```python
from build123d import *

# Parameters (mm, degrees)
SKETCH1_R           = 7.239
SKETCH1_R_2         = 2.15
SKETCH1_R_3         = 1.65
BOSS_EXTRUDE1_DEPTH = 3
FILLET1_R           = 10


with BuildPart() as part:
    # Sketch1 → Boss-Extrude1 (new body)
    with BuildSketch(Plane.XY):
        with BuildLine():
            Line((-87.4, 48.933577685), (87.4, 48.933577685))
            Line((87.4, 48.933577685), (97.4, 48.933577685))
            Line((97.4, 48.933577685), (138.294602876, 18.952308855))
            ThreePointArc((138.294602876, 18.952308855), (147.9, 0), (138.294602876, -18.952308855))
            Line((138.294602876, -18.952308855), (97.4, -48.933577685))
            Line((97.4, -48.933577685), (87.4, -48.933577685))
            Line((87.4, -48.933577685), (-87.4, -48.933577685))
            Line((-87.4, -48.933577685), (-97.4, -48.933577685))
            Line((-97.4, -48.933577685), (-138.294602876, -18.952308855))
            ThreePointArc((-138.294602876, -18.952308855), (-147.9, 0), (-138.294602876, 18.952308855))
            Line((-138.294602876, 18.952308855), (-97.4, 48.933577685))
            Line((-97.4, 48.933577685), (-87.4, 48.933577685))
        make_face()
        with Locations((-87.4, -38)):
            Circle(SKETCH1_R, mode=Mode.SUBTRACT)
        with Locations((-87.4, 38)):
            Circle(SKETCH1_R, mode=Mode.SUBTRACT)
        with Locations((87.4, -38)):
            Circle(SKETCH1_R, mode=Mode.SUBTRACT)
        with Locations((87.4, 38)):
            Circle(SKETCH1_R, mode=Mode.SUBTRACT)
        with Locations((98.110526316, -27)):
            Circle(SKETCH1_R_2, mode=Mode.SUBTRACT)
        with Locations((106.873684211, -18)):
            Circle(SKETCH1_R_2, mode=Mode.SUBTRACT)
        with Locations((106.873684211, 18)):
            Circle(SKETCH1_R_2, mode=Mode.SUBTRACT)
        with Locations((98.110526316, 27)):
            Circle(SKETCH1_R_2, mode=Mode.SUBTRACT)
        with Locations((-98.110526316, -27)):
            Circle(SKETCH1_R_2, mode=Mode.SUBTRACT)
        with Locations((-106.873684211, -18)):
            Circle(SKETCH1_R_2, mode=Mode.SUBTRACT)
        with Locations((-106.873684211, 18)):
            Circle(SKETCH1_R_2, mode=Mode.SUBTRACT)
        with Locations((-98.110526316, 27)):
            Circle(SKETCH1_R_2, mode=Mode.SUBTRACT)
        with Locations((-60, -43.933577685)):
            Circle(SKETCH1_R_3, mode=Mode.SUBTRACT)
        with Locations((0, 43.933577685)):
            Circle(SKETCH1_R_3, mode=Mode.SUBTRACT)
        with Locations((20, 43.933577685)):
            Circle(SKETCH1_R_3, mode=Mode.SUBTRACT)
        with Locations((40, 43.933577685)):
            Circle(SKETCH1_R_3, mode=Mode.SUBTRACT)
        with Locations((60, 43.933577685)):
            Circle(SKETCH1_R_3, mode=Mode.SUBTRACT)
        with Locations((-20, 43.933577685)):
            Circle(SKETCH1_R_3, mode=Mode.SUBTRACT)
        with Locations((-40, 43.933577685)):
            Circle(SKETCH1_R_3, mode=Mode.SUBTRACT)
        with Locations((-60, 43.933577685)):
            Circle(SKETCH1_R_3, mode=Mode.SUBTRACT)
        with Locations((-40, -43.933577685)):
            Circle(SKETCH1_R_3, mode=Mode.SUBTRACT)
        with Locations((-20, -43.933577685)):
            Circle(SKETCH1_R_3, mode=Mode.SUBTRACT)
        with Locations((0, -43.933577685)):
            Circle(SKETCH1_R_3, mode=Mode.SUBTRACT)
        with Locations((20, -43.933577685)):
            Circle(SKETCH1_R_3, mode=Mode.SUBTRACT)
        with Locations((40, -43.933577685)):
            Circle(SKETCH1_R_3, mode=Mode.SUBTRACT)
        with Locations((60, -43.933577685)):
            Circle(SKETCH1_R_3, mode=Mode.SUBTRACT)
    extrude(amount=BOSS_EXTRUDE1_DEPTH)

    # Fillet1
    fillet1_edges = [part.edges().sort_by_distance(p)[0] for p in [
        (-97.4, 48.933577685, 1.5),
        (97.4, 48.933577685, 1.5),
        (97.4, -48.933577685, 1.5),
        (-97.4, -48.933577685, 1.5),
    ]]
    fillet(fillet1_edges, radius=FILLET1_R)


solid = part.part
```
The model under review builds one solid part; all positions refer to its coordinate system, in mm. Give positions to 0.01 mm unless a question says otherwise; leave off trailing zeros. Write each loop counter-clockwise with the first axis right and the second up, starting at its lowest first coordinate (ties: lowest second). Pieces come first, ordered by that corner, then holes. Notation, with made-up numbers: (44.5, 11.25) -> (97.5, 11.25) arc R24 cw to (97.5, 24.25) -> close; hole circle Ø11 at (21.25, -30.75). An arc over 180 degrees is marked (long way). Put each result on its own line as item: value.
(1) We need section B-B, the plane y = -38. Give the boundary of the cut face in (x, z), and give its area (3 significant figures).
Results are:
outline: (-112.31, 0) -> (-94.64, 0) -> (-94.64, 3) -> (-112.31, 3) -> close; (-80.16, 0) -> (80.16, 0) -> (80.16, 3) -> (-80.16, 3) -> close; (94.64, 0) -> (112.31, 0) -> (112.31, 3) -> (94.64, 3) -> close
area: 587 mm²
(2) To check wall thickness, follow probe 1 along Y at (x, z) = (-87.4, 1.1); probe 2 along Y at (x, z) = (-40, 1.55); probe 3 along X at (y, z) = (31.5, 2.1). State the ranges of each line that lie inside material, in increasing order. Write a range as from..to.
Results are:
probe 1: -48.93..-45.24, -30.76..30.76, 45.24..48.93
probe 2: -48.93..-45.58, -42.28..42.28, 45.58..48.93
probe 3: -121.18..-90.59, -84.21..84.21, 90.59..121.18
(3) The part is to be moulded in two halves that separate along Y. For faces 1 (the flat face through (-119.435, 32.779, 1.479)), 2 (the cylindrical face through (85.831, 30.933, 1.479)), 3 (the cylindrical face through (147.9, 0.3, 1.5)), say which applies: pulls with the +Y half, pulls with the -Y half, needs draft (parallel to the pull), parting line crosses it, or undercut.
Results are:
face 1: pulls with the +Y half
face 2: undercut
face 3: parting line crosses it
(4) We need section C-C, the plane z = 0.8. State how many separate pieces and enclosed holes the cut face has, and give its area (3 significant figures).
Results are:
separate pieces: 1
enclosed holes: 26
area: 24,200 mm²
(5) We need section A-A, the plane x = 87.4. Give the boundary of the cut face in (y, z).
Results are:
outline: (-48.93, 0) -> (-45.24, 0) -> (-45.24, 3) -> (-48.93, 3) -> close; (-30.76, 0) -> (30.76, 0) -> (30.76, 3) -> (-30.76, 3) -> close; (45.24, 0) -> (48.93, 0) -> (48.93, 3) -> (45.24, 3) -> close
(6) For pin 1 Ø1 at (y, z) = (8.5, 2) entering from +X, flat-tipped, find the tip position at first contact; note if it passes through.
Results are:
pin 1: x = 146.5
